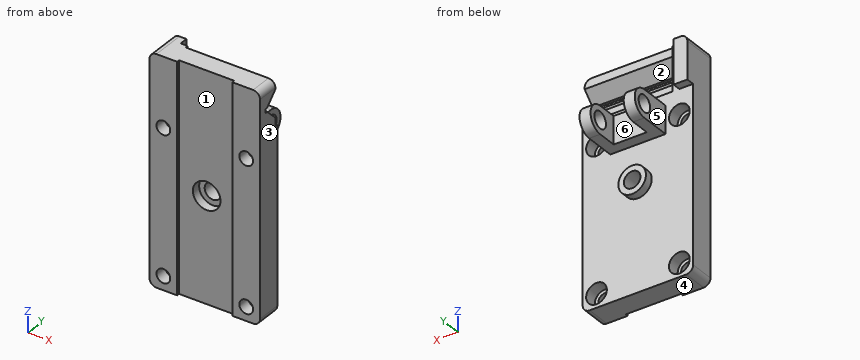
Autodesk Inventor part; units mm, degrees
ref_plane "工作平面1" through (20, 0, 0) normal (1, 0, 0) x (0, 1, 0)
ref_plane "XZ Plane" through (0, 0, 0) normal (0, 1, 0) x (-1, 0, 0)
ref_plane "XY Plane" through (0, 0, 0) normal (0, 0, 1) x (1, 0, 0)
sketch "草图1" plane through (0, 0, 0) normal (0, 1, 0) x (-1, 0, 0)
  line L0 (40, -82) -> (-40, -82)
  line L1 (-40, -82) -> (-40, 82)
  line L2 (-40, 82) -> (40, 82)
  line L3 (40, 82) -> (40, -82)
  line L4 (40, -82) -> (-40, 82) construction
  line L5 (-40, -82) -> (40, 82) construction
  point P0 (0, 0)
  dimension "d0" = 80
  dimension "d1" = 164
extrude "拉伸1" add sketch "草图1" along normal blind 18
sketch "草图2" plane through (0, 18, 0) normal (0, 1, 0) x (1, 0, 0)
  line L0 (-40, -82) -> (40, -82)
  line L1 (-40, 82) -> (-40, -82)
  line L2 (-40, -82) -> (-40, -50)
  line L3 (-40, -50) -> (40, -50)
  line L4 (40, -50) -> (40, -82)
  line L5 (40, -82) -> (-40, -82)
  point P0 (0, 0)
  dimension "d4" = 32
extrude "拉伸2" cut sketch "草图2" against normal blind 2
fillet "圆角1" radius 5 4 edges at (40, 8, 82) (40, 9, -82) (-40, 8, 82) (-40, 9, -82)
sketch "草图4" plane through (0, 0, 0) normal (1, 0, 0) x (0, 1, 0)
  line L0 (0, 82) -> (16, 82)
  line L1 (5.5, 66) -> (5.5, 64.5)
  line L2 (5.5, 64.5) -> (5.5, 67.5)
  line L3 (5.5, 64.5) -> (7.5, 64.5)
  line L4 (7.5, 67.5) -> (5.5, 67.5)
  line L5 (7.5, 64.5) -> (16, 56)
  line L6 (16, 77) -> (16, 50)
  line L7 (7.5, 67.5) -> (16, 76)
  line L8 (16, 76) -> (16, 56)
  line L9 (5.5, 66) -> (6, 66)
  point P0 (0, 0)
  dimension "d15" = 16
  dimension "d16" = 1.5
  dimension "d17" = 3
  dimension "d18" = 2
extrude "拉伸3" cut sketch "草图4" along normal blind 40 and the other way blind 25
sketch "草图6" plane through (0, 16, 0) normal (0, 1, 0) x (1, 0, 0)
  line L0 (40, -76) -> (-25, -76)
  line L1 (-25, -76) -> (-25, -56)
  line L2 (-25, -56) -> (40, -56)
  line L3 (40, -50) -> (40, -56)
  line L4 (-40, -50) -> (40, -50)
  line L5 (-40, -77) -> (-40, -50)
  arc A0 (-40, -77) -> (-35, -82) centre (-35, -77) ccw
  line L6 (35, -82) -> (-35, -82)
  arc A1 (35, -82) -> (40, -77) centre (35, -77) ccw
  line L7 (40, -76) -> (40, -77)
  line L8 (-40, -50) -> (40, -50)
  line L9 (-40, -50) -> (-30, -50)
  line L10 (-30, -50) -> (-30, -82)
  line L11 (-35, -82) -> (35, -82)
  point P0 (0, 0)
  dimension "d27" = 10
extrude "拉伸5" add sketch "草图6" along normal blind 8 contours L6 A0 L5 L4 L10
sketch "草图7" plane through (0, 16, 0) normal (0, 1, 0) x (1, 0, 0)
  line L0 (-30, -50) -> (-30, -82)
  line L1 (35, -82) -> (-30, -82)
  arc A0 (35, -82) -> (40, -77) centre (35, -77) ccw
  line L2 (40, -76) -> (40, -77)
  line L3 (40, -76) -> (-25, -76)
  line L4 (-25, -76) -> (-25, -56)
  line L5 (-25, -56) -> (40, -56)
  line L6 (40, -50) -> (40, -56)
  line L7 (-30, -50) -> (40, -50)
  line L8 (-30, -50) -> (40, -50)
  line L9 (-25, -50) -> (-25, -82)
  line L10 (35, -82) -> (-30, -82)
  point P0 (0, 0)
extrude "拉伸6" add sketch "草图7" along normal blind 2 contours L7 L9 L4 L1 L0
sketch "草图8" plane through (0, 18, 0) normal (0, 1, 0) x (1, 0, 0)
  circle A0 centre (30, -32) radius 7.5
  line L0 (35, -82) -> (-25, -82)
  line L1 (40, -50) -> (40, 77)
  circle A1 centre (30, 72) radius 7.5
  line L2 (35, 82) -> (-35, 82)
  point P0 (0, 0)
  dimension "d32" = 15
  dimension "d34" = 10
  dimension "d35" = 15
  dimension "d36" = 10
  dimension "d38" = 50
extrude "拉伸7" cut sketch "草图8" against normal blind 9
sketch "草图9" plane through (30, 9, -72) normal (0, 1, 0) x (1, 0, 0)
  circle A0 centre (0, 0) radius 7.5
  circle A1 centre (0, -104) radius 7.5
  point P0 (-30, -72)
hole "孔1" at (30, 9, -72) at (30, 9, 32) direction (0, -1, 0) diameter 10 end through all
mirror "镜像1" about plane through (0, 0, 0) normal (1, 0, 0) of "拉伸7", "孔1"
sketch "草图11" plane through (0, 18, 0) normal (0, 1, 0) x (1, 0, 0)
  circle A0 centre (0, 6) radius 10
  line L0 (35, -82) -> (-25, -82)
  point P0 (0, 0)
  dimension "d50" = 20
  dimension "d51" = 88
extrude "拉伸8" add sketch "草图11" along normal blind 6
sketch "草图12" plane through (0, 24, -6) normal (0, 1, 0) x (1, 0, 0)
  circle A0 centre (0, 0) radius 6
  point P0 (0, -6)
  dimension "d54" = 12
extrude "拉伸9" cut sketch "草图12" against normal blind 15.5
sketch "草图13" plane through (0, 0, 0) normal (0, -1, 0) x (1, 0, 0)
  circle A0 centre (-30, -72) radius 5
  circle A1 centre (-30, 32) radius 5
  circle A2 centre (30, -72) radius 5
  circle A3 centre (30, 32) radius 5
  arc A4 (-40, -77) -> (-35, -82) centre (-35, -77) ccw
  line L0 (35, -82) -> (-35, -82)
  arc A5 (35, -82) -> (40, -77) centre (35, -77) ccw
  line L1 (40, 77) -> (40, -77)
  arc A6 (40, 77) -> (35, 82) centre (35, 77) ccw
  line L2 (-35, 82) -> (35, 82)
  arc A7 (-35, 82) -> (-40, 77) centre (-35, 77) ccw
  line L3 (-40, -77) -> (-40, 77)
  circle A8 centre (0, -6) radius 10
  point P0 (0, 0)
  dimension "d57" = 20
  dimension "d58" = 88
extrude "拉伸10" cut sketch "草图13" against normal up to surface (8.5 mm away) contours A8
ref_plane "工作平面1" through (20, 0, 0) normal (1, 0, 0) x (0, 1, 0)
sketch "草图15" plane through (20, 0, 0) normal (1, 0, 0) x (0, 1, 0)
  line L0 (18, 4) -> (18, -16)
  line L1 (18, -64.5) -> (18, -79.5)
  line L2 (18, 39.5) -> (18, 24.5)
  line L3 (18, 39.5) -> (18, 24.5)
  line L4 (18, -64.5) -> (18, -79.5)
  line L5 (18, -77) -> (18, -82)
  line L6 (18, -77) -> (18, 50)
  line L7 (18, 82) -> (18, 50)
  line L8 (18, 82) -> (18, 50)
  line L9 (18, 50) -> (18, -77)
  line L10 (18, -82) -> (18, -77)
  line L11 (18, 39.5) -> (18, 24.5)
  line L12 (16, 82) -> (0, 82)
  line L13 (18, 50) -> (18, -77)
  line L14 (18, 42) -> (40, 42)
  line L15 (40, 22) -> (18, 22)
  line L16 (18, 22) -> (18, 42)
  arc A0 (40, 22) -> (40, 42) centre (40, 32) ccw
  point P0 (0, 0)
  point P1 (18, 32)
  dimension "d62" = 50
  dimension "d63" = 10
  dimension "d66" = 20
  dimension "d67" = 22
extrude "拉伸11" add sketch "草图15" against normal blind 8
sketch "草图16" plane through (12, 0, 0) normal (-1, 0, 0) x (0, 0, 1)
  line L0 (22, 40) -> (22, 18)
  line L1 (22, 18) -> (22, 40)
  line L2 (42, 18) -> (22, 18)
  line L3 (22, 26) -> (42, 26)
  line L4 (42, 26) -> (42, 18)
  line L5 (42, 18) -> (22, 18)
  line L6 (22, 18) -> (22, 26)
  point P0 (0, 0)
  dimension "d70" = 8
extrude "拉伸12" add sketch "草图16" along normal blind 12
sketch "草图17" plane through (20, 0, 0) normal (1, 0, 0) x (0, 0, -1)
  line L0 (-42, 40) -> (-42, 18)
  line L1 (-22, 18) -> (-42, 18)
  line L2 (-22, 18) -> (-22, 40)
  arc A0 (-22, 40) -> (-42, 40) centre (-32, 40) ccw
  circle A1 centre (-32, 40) radius 6
  point P0 (0, 0)
  dimension "d73" = 12
extrude "拉伸13" cut sketch "草图17" against normal blind 8 contours A1
mirror "镜像2" about plane through (0, 0, 0) normal (1, 0, 0) of "拉伸11", "拉伸12", "拉伸13"
sketch "草图18" plane through (0, 0, 0) normal (0, -1, 0) x (1, 0, 0)
  line L0 (12, 22) -> (12, 42)
  circle A0 centre (0, -6) radius 10
  circle A1 centre (-30, -72) radius 5
  circle A2 centre (-30, 32) radius 5
  circle A3 centre (30, -72) radius 5
  circle A4 centre (30, 32) radius 5
  arc A5 (-40, -77) -> (-35, -82) centre (-35, -77) ccw
  line L1 (35, -82) -> (-35, -82)
  arc A6 (35, -82) -> (40, -77) centre (35, -77) ccw
  line L2 (40, 77) -> (40, -77)
  arc A7 (40, 77) -> (35, 82) centre (35, 77) ccw
  line L3 (-35, 82) -> (35, 82)
  arc A8 (-35, 82) -> (-40, 77) centre (-35, 77) ccw
  line L4 (-40, -77) -> (-40, 77)
  line L5 (-35, 82) -> (35, 82)
  line L6 (35, -82) -> (-35, -82)
  line L7 (20, 82) -> (-20, 82)
  line L8 (-20, 82) -> (-20, -82)
  line L9 (-20, -82) -> (20, -82)
  line L10 (20, -82) -> (20, 82)
  point P0 (0, 0)
  dimension "d76" = 20
  dimension "d77" = 40
extrude "拉伸14" cut sketch "草图18" against normal blind 2 contours L8 L3 L10 L1
properties part number "4-上盖" material "灰口铁"
Build history of the part. All positions in model axes, mm. Face numbers are marked on the shaded views. A direction names the side the tool comes from. Coordinates: 2 decimals unless noted, no trailing zeros. Order: outer loops, then holes, each group sorted by start corner. A loop starts at its lowest first (then second) coordinate and runs counter-clockwise, first axis right, second up. Notation, with made-up numbers: (86, -25) -> (123, -25) arc R9 ccw to (123, -14) -> close; hole circle Ø1 at (20.25, 54). An arc over 180 degrees is marked (long way). Answer in a Markdown table with one row per item. Add a question column.
Q1. Band-saw the part on B-B, the plane x = 30. List the corners of the cut face in (y, z).
Q2. Band-saw the part on A-A, the plane z = -6. List the corners of the cut face in (x, y).
Q3. Drop flat-ended pins along their axis: pin 1 (22 mm diameter, centred on x = 0.5, z = -4, fed in from +Y); pin 2 (11 mm diameter, centred on y = 40, z = 32, fed in from -X); pin 3 (6 mm diameter, centred on y = 36.5, z = 36, fed in from +X); pin 4 (17 mm diameter, centred on x = 30, z = -72, fed in from +Y). Give the stop position or say it passes through.
Q4. Mould opens along X. For the marked faces 1, 2 and 3 say: +X half, -X half, draft (parallel to the pull), parting line (faces both ways), or undercut.
Q5. Wall check: line 1 along X through (y, z) = (13, -72); line 2 along Y through (x, z) = (-16.75, 32); line 3 along Z through (x, y) = (-30, 7.25). Give the ranges that are in metal, low to high. Write a range as [from, to].
Q6. Which spindle directions (+Z, -Z, +X, -X, +Y, -Y) get a long thin tool onto all of the face, cutting with end or side? Do the marked faces 4, 5 and 6. Say none if no direction does.
Q7. Band-saw the part on C-C, the plane z = 32. Give the number of separate pieces and of enclosed holes in the cut face, then the cut area to 3 significant figures.
Answers follow:
| question | item | result |
|---|---|---|
| 1 | outline | (0, -82) -> (18, -82) -> (18, -79.5) -> (9, -79.5) -> (9, -77) -> (0, -77) -> close; (0, -67) -> (9, -67) -> (9, -64.5) -> (18, -64.5) -> (18, 24.5) -> (9, 24.5) -> (9, 27) -> (0, 27) -> close; (0, 37) -> (9, 37) -> (9, 39.5) -> (18, 39.5) -> (18, 50) -> (16, 50) -> (16, 56) -> (7.5, 64.5) -> (5.5, 64.5) -> (5.5, 67.5) -> (7.5, 67.5) -> (16, 76) -> (16, 82) -> (0, 82) -> close |
| 2 | outline | (-40, 0) -> (-20, 0) -> (-20, 2) -> (-10, 2) -> (-10, 8.5) -> (-6, 8.5) -> (-6, 24) -> (-10, 24) -> (-10, 18) -> (-40, 18) -> close; (6, 8.5) -> (10, 8.5) -> (10, 2) -> (20, 2) -> (20, 0) -> (40, 0) -> (40, 18) -> (10, 18) -> (10, 24) -> (6, 24) -> close |
| 3 | pin 1 | y = 24 |
| 3 | pin 2 | through |
| 3 | pin 3 | x = 20 |
| 3 | pin 4 | y = 18 |
| 4 | face 1 | undercut |
| 4 | face 2 | draft |
| 4 | face 3 | +X half |
| 5 | line 1 | [-40, -37.5], [-22.5, 22.5], [37.5, 40] |
| 5 | line 2 | [2, 34], [46, 50] |
| 5 | line 3 | [-82, -77], [-67, 27], [37, 82] |
| 6 | face 4 | -Z, +X, -X, +Y, -Y |
| 6 | face 5 | +Z, -Z, -X, +Y |
| 6 | face 6 | +Z, -Z, +Y |
| 7 | separate pieces | 5 |
| 7 | enclosed holes | 0 |
| 7 | area | 1,420 mm^2 |
